```python
from build123d import *

# Parameters (mm, degrees)
BOSS_EXTRUDE1_DEPTH = 14
CUT_EXTRUDE1_REACH  = 94.043
SKETCH2_W           = 11.5
SKETCH2_H           = 8.5
SKETCH3_R           = 1.5
SCREW_HOLES_DEPTH   = 3
SKETCH4_W           = 63
SKETCH4_H           = 8.5
CUT_EXTRUDE2_DEPTH  = 10
CUT_EXTRUDE3_REACH  = 94.043
SKETCH5_W           = 34.745
SKETCH5_H           = 2
SKETCH6_W           = 5.75
SKETCH6_H           = 4
CUT_EXTRUDE4_DEPTH  = 14
BOSS_EXTRUDE2_START = -18.7625
BOSS_EXTRUDE2_DEPTH = 4.7625


with BuildPart() as part:
    # Sketch1 → Boss-Extrude1 (new body)
    with BuildSketch(Plane.XY):
        with BuildLine():
            Line((0, 0), (0, 3))
            Line((0, 3), (8, 3))
            Line((8, 3), (8, 50))
            Line((8, 50), (22, 50))
            ThreePointArc((22, 50), (42, 30), (62, 50))
            Line((62, 50), (76, 50))
            Line((76, 50), (76, 0))
            Line((76, 0), (0, 0))
        make_face()
    extrude(amount=BOSS_EXTRUDE1_DEPTH)

    # Cut-Extrude1: up to this face of the body (flat: up to its plane)
    cut_extrude1_end = Plane(part.part.faces().sort_by_distance((15, 50, 7))[0])
    # Sketch2 → Cut-Extrude1 (cut, up to the picked face)
    with BuildSketch(Plane.XZ, mode=Mode.PRIVATE) as cut_extrude1_sk1:
        with Locations((67.75, 7)):
            Rectangle(SKETCH2_W, SKETCH2_H)
    cut_extrude1_tool1 = split(extrude(cut_extrude1_sk1.sketch, amount=-CUT_EXTRUDE1_REACH, mode=Mode.PRIVATE), bisect_by=cut_extrude1_end, keep=Keep.BOTH, mode=Mode.PRIVATE)
    # Sketch2 → Cut-Extrude1 (cut, up to the picked face)
    with BuildSketch(Plane.XZ, mode=Mode.PRIVATE) as cut_extrude1_sk2:
        with Locations((16.25, 7)):
            Rectangle(SKETCH2_W, SKETCH2_H)
    cut_extrude1_tool2 = split(extrude(cut_extrude1_sk2.sketch, amount=-CUT_EXTRUDE1_REACH, mode=Mode.PRIVATE), bisect_by=cut_extrude1_end, keep=Keep.BOTH, mode=Mode.PRIVATE)
    add(cut_extrude1_tool1.solids().sort_by(Axis((67.75, 0, 7), (0, 1, 0)))[0], mode=Mode.SUBTRACT)
    add(cut_extrude1_tool2.solids().sort_by(Axis((16.25, 0, 7), (0, 1, 0)))[0], mode=Mode.SUBTRACT)

    # Sketch3 → screw holes (cut)
    with BuildSketch(Plane(origin=(0, 3, 0), x_dir=(1, 0, 0), z_dir=(0, 1, 0))):
        with Locations(Location((4, -3, 0), (0, 0, 270))):
            Circle(SKETCH3_R)
        with Locations(Location((4, -11, 0), (0, 0, 270))):
            Circle(SKETCH3_R)
    extrude(amount=-SCREW_HOLES_DEPTH, mode=Mode.SUBTRACT)

    # Sketch4 → Cut-Extrude2 (cut)
    with BuildSketch(Plane(origin=(0, 50, 0), x_dir=(1, 0, 0), z_dir=(0, 1, 0))):
        with Locations((42, -7)):
            Rectangle(SKETCH4_W, SKETCH4_H)
    extrude(amount=-CUT_EXTRUDE2_DEPTH, mode=Mode.SUBTRACT)

    # Cut-Extrude3: up to this face of the body (flat: up to its plane)
    cut_extrude3_end = Plane(part.part.faces().sort_by_distance((41.673782579, 21.087311786, 14))[0])
    # Sketch5 → Cut-Extrude3 (cut, up to the picked face)
    with BuildSketch(Plane(origin=(0, 0, 0), x_dir=(-1, 0, 0), z_dir=(0, 0, -1)), mode=Mode.PRIVATE) as cut_extrude3_sk1:
        with Locations((-58.6275, 1)):
            Rectangle(SKETCH5_W, SKETCH5_H)
    cut_extrude3_tool1 = split(extrude(cut_extrude3_sk1.sketch, amount=-CUT_EXTRUDE3_REACH, mode=Mode.PRIVATE), bisect_by=cut_extrude3_end, keep=Keep.BOTH, mode=Mode.PRIVATE)
    add(cut_extrude3_tool1.solids().sort_by(Axis((58.6275, 1, 0), (0, 0, 1)))[0], mode=Mode.SUBTRACT)

    # Sketch6 → Cut-Extrude4 (cut)
    with BuildSketch(Plane.XY.offset(14)):
        with Locations((44.43, 4)):
            Rectangle(SKETCH6_W, SKETCH6_H)
    extrude(amount=-CUT_EXTRUDE4_DEPTH, mode=Mode.SUBTRACT)

    # Sketch7 → Boss-Extrude2 (add)
    with BuildSketch(Plane.XY.offset(14).offset(BOSS_EXTRUDE2_START)):
        with BuildLine():
            Line((22, 50), (20, 50))
            ThreePointArc((20, 50), (42, 28), (64, 50))
            Line((64, 50), (62, 50))
            ThreePointArc((62, 50), (42, 30), (22, 50))
        make_face()
    extrude(amount=BOSS_EXTRUDE2_DEPTH)


solid = part.part
```
Here's how the part is built. I have some questions about the finished solid (model axes, mm). A direction names the side the tool comes from. Round coordinates to 2 decimals unless told otherwise and drop trailing zeros. Loops run counter-clockwise (first coordinate to the right, second up) from the corner with the lowest first, then second, coordinate; pieces in that order, holes last.
1. Suppose I cut it at B-B, the plane x = 4. Please give me the cut outline in (y, z), and give its area (3 significant figures).
Answers:
outline: (0, 0) - (3, 0) - (3, 1.5) - (0, 1.5) - close; (0, 4.5) - (3, 4.5) - (3, 9.5) - (0, 9.5) - close; (0, 12.5) - (3, 12.5) - (3, 14) - (0, 14) - close
area: 24.0 mm2
2. Suppose I cut it at C-C, the plane z = 7.5. Give the number of separate pieces and of enclosed holes in the cut face, and give its area (3 significant figures).
Answers:
separate pieces: 3
enclosed holes: 0
area: 1,560 mm2
3. Suppose I cut it at D-D, the plane y = 44. Please give me the cut outline in (x, z).
Answers:
outline: (8, 0) - (20.83, 0) - (20.83, -4.76) - (22.92, -4.76) - (22.92, 2.75) - (10.5, 2.75) - (10.5, 11.25) - (22.92, 11.25) - (22.92, 14) - (8, 14) - close; (61.08, -4.76) - (63.17, -4.76) - (63.17, 0) - (76, 0) - (76, 14) - (61.08, 14) - (61.08, 11.25) - (73.5, 11.25) - (73.5, 2.75) - (61.08, 2.75) - close
4. For faces 5 (the face through (41.555, 4, 7)), 6 (the face through (59, 2, 7)), 7 (the face through (42, 28, -2)), 8 (the face through (10.5, 25, 7)), which set-ups out of +Z, -Z, +X, -X, +Y, -Y let a thin tool reach every point of the face, with its end or its side?
Answers:
face 5: +Z, -Z, -Y
face 6: +Z, -Z, +X, -Y
face 7: -Z, -Y
face 8: +Y, -Y
5. If I drill on probe 1 along X at (y, z) = (2.1, 11) (3 decimals); probe 2 along X at (y, z) = (15.5, 3.25); probe 3 along X at (y, z) = (1.45, 11) (3 decimals), over which ranges is the centre line in solid material (lowest first)?
Answers:
probe 1: x = 0 to 2.5, 5.5 to 10.5, 22 to 41.555, 47.305 to 62, 73.5 to 76
probe 2: x = 8 to 10.5, 22 to 62, 73.5 to 76
probe 3: x = 0 to 2.5, 5.5 to 10.5, 22 to 41.255
6. Suppose I cut it at A-A, the plane y = 10. Please give me the cut outline in (x, z), and give its area (4 significant figures).
Answers:
outline: (8, 0) - (76, 0) - (76, 14) - (8, 14) - close; hole (10.5, 2.75) - (22, 2.75) - (22, 11.25) - (10.5, 11.25) - close; hole (62, 2.75) - (73.5, 2.75) - (73.5, 11.25) - (62, 11.25) - close
area: 756.5 mm2
7. Thinking about a two-plate mould opening in Z: for faces 1 (the face through (4, 3, 7)), 2 (the face through (62, 21, 7)), 3 (the face through (22, 20, 7)), 4 (the face through (47, 20, 0)), which applies, released by +Z, released by -Z, zero draft, split by the parting line, or undercut?
Answers:
face 1: zero draft
face 2: undercut
face 3: undercut
face 4: released by -Z
8. Will these pins go through, and if not, where does the flat tip stop? pin 1 (8 mm diameter, centred on x = 54, z = 11, fed in from -Y); pin 2 (4.5 mm diameter, centred on x = 17.5, y = 29, fed in from -Z); pin 3 (4 mm diameter, centred on y = 19.5, z = 9, fed in from -X); pin 4 (2.5 mm diameter, centred on x = 4, z = 3, fed in from +Y).
Answers:
pin 1: stops at y = 2
pin 2: stops at z = 0
pin 3: stops at x = 8
pin 4: passes through
